Work out the finished part from the listing and answer in its coordinate system (mm). Face numbers are marked on the shaded views. A direction names the side the tool comes from. Give positions to 0.01 mm unless a question says otherwise; leave off trailing zeros. Loops run counter-clockwise (first coordinate to the right, second up) from the corner with the lowest first, then second, coordinate; pieces in that order, holes last. Notation, with made-up numbers: (71, 53) -> (82, 53) arc R37 cw to (82, 91) -> close; hole circle Ø11 at (-16, 78). An arc over 180 degrees is marked (long way). Answer as CSV lines item,"result". Start each with the question number.
1. Find section B-B, the plane x = -68.58. Give the vertices of the cut face in (y, z), and give its area (3 significant figures).
2. Find the intervals of material crossed by line 1 along X through (y, z) = (-68, -7); line 2 along Y through (x, z) = (-68, 26); line 3 along Z through (x, y) = (-25, -56), in increasing order.
3. Find section D-D, the plane x = -21.5. Give the vertices of the cut face in (y, z).
4. Find section A-A, the plane z = -17.78. Give the vertices of the cut face in (x, y), and give its area (3 significant figures).
5. Determine the mould class of the marked faces 4, 5, 6 and 7 for opening direction Z: +Z half, -Z half, draft (parallel to the pull), parting line (faces both ways), or undercut.
6. Flat-ended cylindrical pins translate along their axes: pin 1 Ø3 at (y, z) = (-91, -36.5) entering from +X; pin 2 Ø10 at (x, y) = (-24, -105) entering from -Z; pin 3 Ø1 at (y, z) = (-66, 47.5) entering from +X. Find the tip coordinate at first contact, or state that the pin passes through.
7. Find section C-C, the plane y = -16.5. Give the vertices of the cut face in (x, z), and give its area (3 significant figures).
8. A tool of negligible diameter and unlimited length cuts with its end or side. For the marked faces 1, 2 and 3, from which of +Z, -Z, +X, -X, +Y, -Y can it reach the whole face along a straight path? Write none if from no direction.
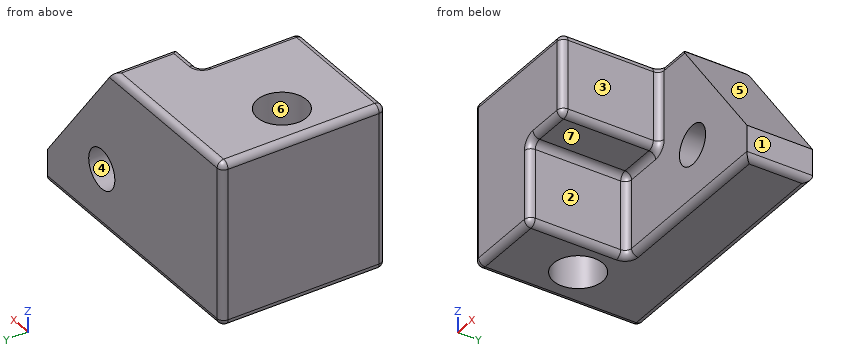
from build123d import *

# Parameters (mm, degrees)
F0_W        = 203.2
F0_H        = 127
F1_DEPTH    = 127
F3_DEPTH    = 25.4
F4_DEPTH    = 101.6
F5_T1_DEPTH = 575.1977482789
F6_R        = 5.08
F7_R        = 15.24
F8_DEPTH    = 50.8
F9_R        = 19.05
F10_DEPTH   = 127


# Not quite as in the source:
# - a fillet or chamfer that OpenCascade refuses, or shapes differently, is made with other operations: its cross-section is extruded or revolved along the edge and cut away or added


with BuildPart() as f1:
    # F0 (on Front) → F1 (new body)
    with BuildSketch(Plane.XZ):
        Rectangle(F0_W, F0_H)
    extrude(amount=F1_DEPTH)

    # F2 (on face) → F3 (join)
    with BuildSketch(Plane.XZ.offset(127)):
        Polygon((101.6, 63.5), (0, 63.5), (0, 0), (-38.1, 0), (-38.1, -63.5), (101.6, -63.5), align=None)
    extrude(amount=F3_DEPTH)

    # F4 (cut): a face of the model
    f4_faces = [f1.faces().sort_by_distance(p)[0] for p in [
        (39.7710526316, -152.4, -5.0131578947),
    ]]
    extrude(f4_faces, amount=-F4_DEPTH, mode=Mode.SUBTRACT)

    # F5: chamfer of 76.2 x 101.6 on 1 edges, made by hand

    # F5_s2 → F5_t1 (cut)
    with BuildSketch(Plane.XZ.offset(-262.1988741395)):
        Polygon((101.6, -38.1), (25.4, 63.5), (101.6, 63.5), align=None)
    extrude(amount=F5_T1_DEPTH, mode=Mode.SUBTRACT)

    # F6
    f6_edges = [f1.edges().sort_by_distance(p)[0] for p in [
        (-50.8, -127, 63.5),
        (0, -88.9, 63.5),
        (0, -127, 31.75),
        (-19.05, -127, 0),
        (-69.85, -127, -63.5),
        (-101.6, -127, 0),
        (-38.1, -127, -31.75),
        (-38.1, -88.9, -63.5),
        (31.75, -50.8, -63.5),
        (-38.1, -50.8, -31.75),
        (101.6, -25.4, -63.5),
        (0, 0, -63.5),
        (-101.6, 0, 0),
        (-101.6, -63.5, -63.5),
        (12.7, -50.8, 63.5),
        (25.4, -25.4, 63.5),
        (-38.1, 0, 63.5),
        (0, -88.9, 0),
        (-19.05, -50.8, 0),
        (-38.1, -88.9, 0),
        (-101.6, -63.5, 63.5),
        (0, -50.8, 31.75),
    ]]
    fillet(f6_edges, radius=F6_R)

    # F7 (on face) → F8 (cut, through all)
    with BuildSketch(Plane.XZ.offset(50.8)):
        with Locations((38.1, -17.78)):
            Circle(F7_R)
    extrude(amount=-F8_DEPTH, mode=Mode.SUBTRACT)

    # F9 (on face) → F10 (cut, through all)
    with BuildSketch(Plane.XY.offset(63.5)):
        with Locations((-68.58, -68.58)):
            Circle(F9_R)
    extrude(amount=-F10_DEPTH, mode=Mode.SUBTRACT)


solid = f1.part
Resolved:
1,outline,"(-127, -58.42) arc R5.08 ccw to (-121.92, -63.5) -> (-87.63, -63.5) -> (-87.63, 63.5) -> (-121.92, 63.5) arc R5.08 ccw to (-127, 58.42) -> close; (-49.53, -63.5) -> (-5.08, -63.5) arc R5.08 ccw to (0, -58.42) -> (0, 58.42) arc R5.08 ccw to (-5.08, 63.5) -> (-49.53, 63.5) -> close"
1,area,"11,300 mm^2"
2,line 1,"x = -101.6 to -87.62, -49.54 to -38.1"
2,line 2,"y = -127 to -87.62, -49.54 to 0"
2,line 3,"z = 0 to 63.5"
3,outline,"(-127, 5.08) arc R5.08 ccw to (-121.92, 0) -> (-55.88, 0) arc R5.08 cw to (-50.8, -5.08) -> (-50.8, -58.42) arc R5.08 ccw to (-45.72, -63.5) -> (-5.08, -63.5) arc R5.08 ccw to (0, -58.42) -> (0, 58.42) arc R5.08 ccw to (-5.08, 63.5) -> (-121.92, 63.5) arc R5.08 ccw to (-127, 58.42) -> close"
4,outline,"(-101.6, -121.92) arc R5.08 ccw to (-96.52, -127) -> (-43.18, -127) arc R5.08 ccw to (-38.1, -121.92) -> (-38.1, -55.88) arc R5.08 cw to (-33.02, -50.8) -> (22.86, -50.8) -> (22.86, 0) -> (-96.52, 0) arc R5.08 ccw to (-101.6, -5.08) -> close; (53.34, -50.8) -> (86.36, -50.8) -> (86.36, 0) -> (53.34, 0) -> close; hole circle Ø38.1 at (-68.58, -68.58)"
4,area,"11,700 mm^2"
5,face 4,"undercut"
5,face 5,"+Z half"
5,face 6,"draft"
5,face 7,"-Z half"
6,pin 1,"stops at x = -38.1"
6,pin 2,"stops at z = 0"
6,pin 3,"stops at x = 0"
7,outline,"(-101.6, -58.42) arc R5.08 ccw to (-96.52, -63.5) -> (96.52, -63.5) arc R5.08 ccw to (101.6, -58.42) -> (101.6, -38.1) -> (26.92, 61.47) arc R5.08 ccw to (22.86, 63.5) -> (-96.52, 63.5) arc R5.08 ccw to (-101.6, 58.42) -> close; hole circle Ø30.48 at (38.1, -17.78)"
7,area,"21,200 mm^2"
8,face 1,"+Z, -Z, +X, +Y, -Y"
8,face 2,"-Z, +X, -Y"
8,face 3,"+Z, -Z, +X, -Y"
